```python
from build123d import *

# Parameters (mm, degrees)
SKETCH1_W           = 70
SKETCH1_H           = 20
BOSS_EXTRUDE1_DEPTH = 8
CUT_EXTRUDE1_DEPTH  = 74.239333694
FILLET1_R           = 0.5
FILLET2_R           = 0.5


with BuildPart() as part:
    # Sketch1 → Boss-Extrude1 (new body)
    with BuildSketch(Plane.XY):
        with Locations((35, 10)):
            Rectangle(SKETCH1_W, SKETCH1_H)
    extrude(amount=BOSS_EXTRUDE1_DEPTH)

    # Sketch2 → Cut-Extrude1 (cut, through all)
    with BuildSketch(Plane(origin=(70, 0, 0), x_dir=(0, 0, -1), z_dir=(1, 0, 0))):
        Polygon((-8, 6), (-6.5, 6), (-2.5, 3), (-2.5, 17), (-6.5, 14), (-8, 14), align=None)
    extrude(amount=-CUT_EXTRUDE1_DEPTH, mode=Mode.SUBTRACT)

    # Fillet1
    fillet1_edges = [part.edges().sort_by_distance(p)[0] for p in [
        (35, 3, 2.5),
    ]]
    fillet(fillet1_edges, radius=FILLET1_R)

    # Fillet2
    fillet2_edges = [part.edges().sort_by_distance(p)[0] for p in [
        (35, 17, 2.5),
    ]]
    fillet(fillet2_edges, radius=FILLET2_R)


solid = part.part
```
Geometry: final body of the model. Coordinates: model frame, mm. A direction names the side the tool comes from. Give positions to 0.01 mm unless a question says otherwise; leave off trailing zeros. Write each loop counter-clockwise with the first axis right and the second up, starting at its lowest first coordinate (ties: lowest second). Pieces come first, ordered by that corner, then holes.
1. Reachability of faces 5 (the flat face through (35, 14, 7)), 6 (the flat face through (70, 10, 2)), 7 (the flat face through (35.5, 4.8, 4.9)) from +Z, -Z, +X, -X, +Y, -Y: full face, straight path, thin tool, end or side. Return the list, or none.
2. Line query: probe 1 along Y at (x, z) = (37, 7.25); probe 2 along Z at (x, y) = (59.5, 11.5); probe 3 along Y at (x, z) = (11, 3.25). Output: solid intervals per line, ascending.
3. Section query B-B, the plane x = 8. Return loops of the section in (y, z).
4. Draft query along Z for faces 1 (the flat face through (35, 3, 8)), 2 (the flat face through (35, 10, 0)), 3 (the flat face through (35.5, 15.2, 4.9)), 4 (the flat face through (35, 0, 4)). Return one class per face: released by +Z, released by -Z, zero draft, split by the parting line, or undercut.
5. Section query A-A, the plane z = 4.25. Return loops of the section in (x, y), then the cut area to 3 significant figures.
6. Section query C-C, the plane y = 7.25. Return loops of the section in (x, z), then the cut area to 3 significant figures.
7. Pin query (flat end, axial travel): P1, Ø12, axis at x = 17, y = 13.5, coming from the +Z side. Return the tip coordinate at first contact, or that it passes through.
Computed:
1. face 5: +Z, +X, -X
1. face 6: +Z, -Z, +X, +Y, -Y
1. face 7: +X, -X
2. probe 1: y = 0 to 6, 14 to 20
2. probe 2: z = 0 to 2.5
2. probe 3: y = 0 to 3.57, 16.43 to 20
3. outline: (0, 0) - (20, 0) - (20, 8) - (14, 8) - (14, 6.5) - (16.4, 3.3) arc R0.5 cw to (16, 2.5) - (4, 2.5) arc R0.5 cw to (3.6, 3.3) - (6, 6.5) - (6, 8) - (0, 8) - close
4. face 1: released by +Z
4. face 2: released by -Z
4. face 3: undercut
4. face 4: zero draft
5. outline: (0, 0) - (70, 0) - (70, 4.31) - (0, 4.31) - close; (0, 15.69) - (70, 15.69) - (70, 20) - (0, 20) - close
5. area: 604 mm2
6. outline: (0, 0) - (70, 0) - (70, 2.5) - (0, 2.5) - close
6. area: 175 mm2
7. P1: stops at z = 8
